Check sheet for the modelled part. Datum: model origin and axes. Units: mm. A direction names the side the tool comes from. Round coordinates to 2 decimals unless told otherwise and drop trailing zeros. Write each loop counter-clockwise with the first axis right and the second up, starting at its lowest first coordinate (ties: lowest second). Pieces come first, ordered by that corner, then holes. Notation, with made-up numbers: (19.5, 3) -> (74.5, 3) arc R21 cw to (74.5, 23) -> close; hole circle Ø4 at (32, 53.25). An arc over 180 degrees is marked (long way). Answer as a JSON object with one key per item and string values. Group by question number.
```python
from build123d import *

# Parameters (mm, degrees)
F0_W     = 84
F0_H     = 21
F0_W_2   = 78
F0_H_2   = 3
F0_W_3   = 72
F0_R     = 1.5
F1_DEPTH = 2
F2_R     = 1
F3_R     = 1.5
F4_DEPTH = 2
F5_R     = 10
F6_R     = 4.49999


# Not quite as in the source:
# - a fillet or chamfer is up to 0.001 mm smaller than in the source, because OpenCascade refuses the exact size


with BuildPart() as f1:
    # F0 (on Front) → F1 (new body)
    with BuildSketch(Plane.XZ):
        Rectangle(F0_W, F0_H)
        with Locations((0, -6)):
            Rectangle(F0_W_2, F0_H_2, mode=Mode.SUBTRACT)
        with Locations((-3, 6)):
            Rectangle(F0_W_3, F0_H_2, mode=Mode.SUBTRACT)
        with Locations((37.5, 6)):
            Circle(F0_R, mode=Mode.SUBTRACT)
    extrude(amount=F1_DEPTH)

    # F2
    f2_edges = [f1.edges().sort_by_distance(p)[0] for p in [
        (-39, -1, 7.5),
        (-39, -1, -4.5),
        (-39, -1, 4.5),
        (-39, -1, -7.5),
        (33, -1, 7.5),
        (39, -1, -4.5),
        (39, -1, -7.5),
        (33, -1, 4.5),
    ]]
    fillet(f2_edges, radius=F2_R)

    # F3 (on face) → F4 (join)
    with BuildSketch(Plane.XZ.offset(2)):
        Polygon((-42, -10.5), (-42, 0), (-42, 10.5), (-49, 10.5), (-49, 32.5), (-58, 32.5), (-58, -10.5), align=None)
        with Locations((-53.5, 3)):
            Circle(F3_R, mode=Mode.SUBTRACT)
        with Locations((-53.5, 28)):
            Circle(F3_R, mode=Mode.SUBTRACT)
        Polygon((42, 10.5), (42, 0), (42, -10.5), (58, -10.5), (58, 32.5), (49, 32.5), (49, 10.5), align=None)
        with Locations((53.5, 3)):
            Circle(F3_R, mode=Mode.SUBTRACT)
        with Locations((53.5, 28)):
            Circle(F3_R, mode=Mode.SUBTRACT)
    extrude(amount=-F4_DEPTH)

    # F5
    f5_edges = [f1.edges().sort_by_distance(p)[0] for p in [
        (-49, -1, 10.5),
        (49, -1, 10.5),
    ]]
    fillet(f5_edges, radius=F5_R)

    # F6 (radius 4.5 in the source; OpenCascade refuses exactly that, so slightly less here)
    f6_edges = [f1.edges().sort_by_distance(p)[0] for p in [
        (-49, -1, 32.5),
        (-58, -1, 32.5),
        (58, -1, 32.5),
        (49, -1, 32.5),
    ]]
    fillet(f6_edges, radius=F6_R)


solid = f1.part
```
(1) Go/stop test with flat-tipped pins: pin 1 Ø4 at (x, z) = (53.5, 28) entering from +Y; pin 2 Ø0.6 at (x, y) = (4, -1.5) entering from +Z; pin 3 Ø2.5 at (x, z) = (-53.5, 3) entering from -Y. Record where each tip stops, or that it passes through.
(2) Section check A-A on x = -23.5. Record the cut outline in (y, z).
(3) Section check D-D on x = -43. Record the cut outline in (y, z).
(4) Scan lines: line 1 along Z through (x, y) = (53.5, -1.3); line 2 along Z through (x, y) = (13, -0.7); line 3 along Z through (x, y) = (35, -0.45). Record each from-to range of solid material in increasing order.
(5) Release check for a two-part mould opening along X. For faces 1 (the flat face through (-49, -1, 24)), 2 (the cylindrical face through (50.283, -0.986, 31.147)), 3 (the flat face through (58, -1, 8)), 4 (the flat face through (-1, 0, 2)) record: pulls with the +X half, pulls with the -X half, needs draft (parallel to the pull), parting line crosses it, or undercut.
(6) Section check B-B on z = 3. Record the cut outline in (x, y).
(7) Access from +Z, -Z, +X, -X, +Y, -Y to the whole of each face (thin tool, end or side, straight path). Record for faces 5 (the cylindrical face through (56.647, -0.986, 31.217)), 6 (the cylindrical face through (-46.15, -0.99, 13.51)), 7 (the flat face through (-3, -1, 7.5)).
(8) Section check C-C on y = -1.1. State how many separate pieces and enclosed holes the cut face has, then the cut area to 3 significant figures.
Data:
{
 "1": {"pin 1": "stops at y = 0", "pin 2": "stops at z = 10.5", "pin 3": "passes through"},
 "2": {"outline": "(-2, -10.5) -> (0, -10.5) -> (0, -7.5) -> (-2, -7.5) -> close; (-2, -4.5) -> (0, -4.5) -> (0, 4.5) -> (-2, 4.5) -> close; (-2, 7.5) -> (0, 7.5) -> (0, 10.5) -> (-2, 10.5) -> close"},
 "3": {"outline": "(-2, -10.5) -> (0, -10.5) -> (0, 11.33) -> (-2, 11.33) -> close"},
 "4": {"line 1": "z = -10.5 to 1.5, 4.5 to 26.5, 29.5 to 32.5", "line 2": "z = -10.5 to -7.5, -4.5 to 4.5, 7.5 to 10.5", "line 3": "z = -10.5 to -7.5, -4.5 to 10.5"},
 "5": {"face 1": "undercut", "face 2": "undercut", "face 3": "pulls with the +X half", "face 4": "needs draft"},
 "6": {"outline": "(-58, -2) -> (-55, -2) -> (-55, 0) -> (-58, 0) -> close; (-52, -2) -> (52, -2) -> (52, 0) -> (-52, 0) -> close; (55, -2) -> (58, -2) -> (58, 0) -> (55, 0) -> close"},
 "7": {"face 5": "+Z, +X, +Y, -Y", "face 6": "+Z, +Y, -Y", "face 7": "+Y, -Y"},
 "8": {"separate pieces": "1", "enclosed holes": "7", "area": "2,370 mm²"}
}
